```python
from build123d import *

# Parameters (mm, degrees)
SKETCH_1_R          = 1.5
EXTRUDE_1_DEPTH     = 5
CUT_EXTRUDE_1_DEPTH = 84.692683778


with BuildPart() as part:
    # 스케치1 → 보스-돌출1 (new body)
    with BuildSketch(Plane.XY):
        with BuildLine():
            Line((20.05, 5), (0, 5))
            ThreePointArc((0, 5), (-5, 0), (0, -5))
            Line((0, -5), (22, -5))
            Line((22, -5), (26.601353767, 1.956410875))
            Line((26.601353767, 1.956410875), (36.025134241, 5.963228766))
            Line((36.025134241, 5.963228766), (42.488975113, 3.018953392))
            Line((42.488975113, 3.018953392), (43.498164032, 3.018953392))
            Line((43.498164032, 3.018953392), (44.062133892, 4.253931713))
            Line((44.062133892, 4.253931713), (45.402427297, 4.470373499))
            Line((45.402427297, 4.470373499), (46.008680673, 5.685153438))
            Line((46.008680673, 5.685153438), (47.107948843, 5.685153438))
            Line((47.107948843, 5.685153438), (47.498446434, 6.712724429))
            Line((47.498446434, 6.712724429), (48.640951743, 6.712724429))
            Line((48.640951743, 6.712724429), (49.103035082, 7.757615508))
            Line((49.103035082, 7.757615508), (50.245112942, 7.726365831))
            Line((50.245112942, 7.726365831), (50.735603144, 8.758227131))
            Line((50.735603144, 8.758227131), (51.876398977, 8.69575116))
            Line((51.876398977, 8.69575116), (52.394929025, 9.713810574))
            Line((52.394929025, 9.713810574), (53.533589213, 9.620155058))
            Line((53.533589213, 9.620155058), (54.079771108, 10.623650806))
            Line((54.079771108, 10.623650806), (55.215443631, 10.498885825))
            Line((55.215443631, 10.498885825), (55.788868685, 11.487067026))
            Line((55.788868685, 11.487067026), (56.920703758, 11.331285936))
            Line((56.920703758, 11.331285936), (57.520942896, 12.303413169))
            Line((57.520942896, 12.303413169), (58.648093605, 12.116732536))
            Line((58.648093605, 12.116732536), (59.274697688, 13.072078391))
            Line((59.274697688, 13.072078391), (60.396320625, 12.854637901))
            Line((60.396320625, 12.854637901), (61.048820788, 13.792487525))
            Line((61.048820788, 13.792487525), (62.164076682, 13.544449883))
            Line((62.164076682, 13.544449883), (62.84198468, 14.464101515))
            Line((62.84198468, 14.464101515), (63.950039022, 14.185652318))
            Line((63.950039022, 14.185652318), (64.652847601, 15.086417815))
            Line((64.652847601, 15.086417815), (65.752871272, 14.777765417))
            Line((65.752871272, 14.777765417), (66.480054544, 15.658970767))
            Line((66.480054544, 15.658970767), (67.571224435, 15.320346122))
            Line((67.571224435, 15.320346122), (68.322238273, 16.181331949))
            Line((68.322238273, 16.181331949), (69.403737898, 15.812988438))
            Line((69.403737898, 15.812988438), (70.165521035, 16.650113087))
            Line((70.165521035, 16.650113087), (71.224188399, 16.249719983))
            Line((71.224188399, 16.249719983), (72.008283749, 17.065983242))
            Line((72.008283749, 17.065983242), (73.055761076, 16.637168043))
            Line((73.055761076, 16.637168043), (73.861597574, 17.431975419))
            Line((73.861597574, 17.431975419), (74.897121975, 16.975050435))
            Line((74.897121975, 16.975050435), (75.724112721, 17.74782306))
            Line((75.724112721, 17.74782306), (76.746930013, 17.263121075))
            Line((76.746930013, 17.263121075), (77.594472701, 18.013296132))
            Line((77.594472701, 18.013296132), (78.603837954, 17.501170159))
            Line((78.603837954, 17.501170159), (79.484104239, 18.229489901))
            Line((79.484104239, 18.229489901), (77.772918882, 22.391441928))
            Line((77.772918882, 22.391441928), (70.455863435, 25.724355994))
            Line((70.455863435, 25.724355994), (20.05, 5))
        make_face()
        with Locations((35.039512437, 8.36046215)):
            Circle(SKETCH_1_R, mode=Mode.SUBTRACT)
        Circle(SKETCH_1_R, mode=Mode.SUBTRACT)
        with Locations((22, 0)):
            Circle(SKETCH_1_R, mode=Mode.SUBTRACT)
        with Locations((67.410250422, 21.669681595)):
            Circle(SKETCH_1_R, mode=Mode.SUBTRACT)
    extrude(amount=EXTRUDE_1_DEPTH)

    # 스케치2 → 컷-돌출1 (cut, through all)
    with BuildSketch(Plane.XY.offset(5)):
        with BuildLine():
            Line((26.601353767, 1.956410875), (24.524988327, 6.83989014))
            Line((24.524988327, 6.83989014), (20.05, 5))
            Line((20.05, 5), (0, 5))
            ThreePointArc((0, 5), (-5, 0), (0, -5))
            Line((0, -5), (22, -5))
            Line((22, -5), (26.601353767, 1.956410875))
        make_face()
    extrude(amount=-CUT_EXTRUDE_1_DEPTH, mode=Mode.SUBTRACT)


solid = part.part
```
Check sheet for the modelled part. Datum: model origin and axes. Units: mm. A direction names the side the tool comes from. Coordinates: 2 decimals unless noted, no trailing zeros. Order: outer loops, then holes, each group sorted by start corner. A loop starts at its lowest first (then second) coordinate and runs counter-clockwise, first axis right, second up. Notation, with made-up numbers: M -8.75,5 L 47.25,5 A28 ccw 47.25,25 Z; hole C -0.75,-39.75 d5. An arc over 180 degrees is marked long. One line per question, with ' | ' between items. Start each with the question number.
Item 1: Mould release check, pull along X, two halves, no side actions. Record for faces 3 (the flat face through (63.388, 14.327, 2.465)), 4 (the flat face through (43, 3.019, 2)), 5 (the flat face through (74.166, 24.035, 2.465)): pulls with the +X half, pulls with the -X half, needs draft (parallel to the pull), parting line crosses it, or undercut.
Item 2: Material ranges on line 1 (X direction, y = 7.5, z = 3.45); line 2 (X direction, y = 22.5, z = 3.75); line 3 (Y direction, x = 37, z = 4.1), recorded low to high.
Item 3: Sectioned sample at C-C on y = 19.5. Record the cut outline in (x, z), and give its area (3 significant figures).
Item 4: Sectioned sample at B-B on z = 1.9. Count the separate pieces of the cut face and the enclosed holes in it, and give its area (3 significant figures).
Item 5: Access from +Z, -Z, +X, -X, +Y, -Y to the whole of each face (thin tool, end or side, straight path). Record for faces 1 (the flat face through (62.5, 14, 2.5)), 2 (the flat face through (47.3, 6.19, 2.46)).
Item 6: Gauge pin test, flat ends, axial feed: P1, Ø1.5, axis at x = 39.5, z = 1, coming from the -Y side; P2, Ø5, axis at x = 60.5, y = 11, coming from the +Z side; P3, Ø1.5, axis at y = 20.5, z = 2.5, coming from the -X side (3 decimals); P4, Ø1, axis at x = 67, z = 4, coming from the +Y side. Record the tip position at first contact, or that the pin passes through.
Item 7: Sectioned sample at A-A on x = 40.5. Record the cut outline in (y, z), and give its area (3 significant figures).
Answer below:
1) face 3: undercut | face 4: needs draft | face 5: pulls with the +X half
2) line 1: x = 26.13 to 33.81, 36.27 to 48.99 | line 2: x = 62.61 to 66.16, 68.66 to 77.53 | line 3: y = 5.52 to 11.97
3) outline: M 55.32,0 L 78.96,0 L 78.96,5 L 55.32,5 Z | area: 118 mm^2
4) separate pieces: 1 | enclosed holes: 2 | area: 411 mm^2
5) face 1: +Z, -Z, -Y | face 2: +Z, -Z, +X, -Y
6) P1: stops at y = 4.04 | P2: stops at z = 5 | P3: stops at x = 55.925 | P4: stops at y = 24.51
7) outline: M 3.92,0 L 13.41,0 L 13.41,5 L 3.92,5 Z | area: 47.4 mm^2
